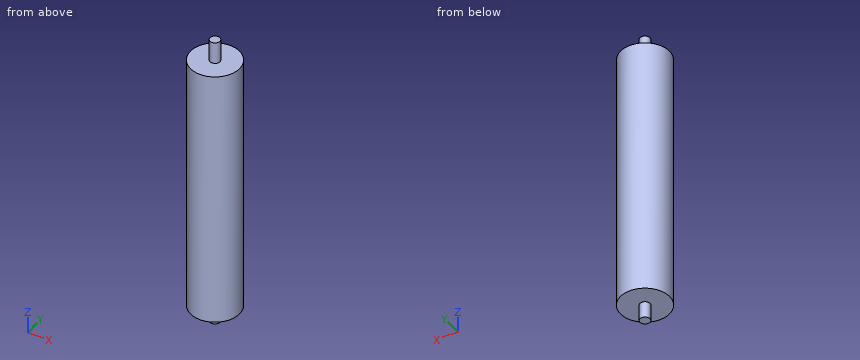
Autodesk Inventor part; units mm, degrees
ref_plane "YZ Plane" through (0, 0, 0) normal (1, 0, 0) x (0, 1, 0)
ref_plane "XZ Plane" through (0, 0, 0) normal (0, 1, 0) x (-1, 0, 0)
ref_plane "XY Plane" through (0, 0, 0) normal (0, 0, 1) x (1, 0, 0)
sketch "草图1" plane through (0, 0, 0) normal (0, 0, 1) x (1, 0, 0)
  circle A0 centre (0, 0) radius 4.6
  dimension "d0" = 9.2
extrude "拉伸1" add sketch "草图1" along normal blind 20
sketch "草图2" plane through (0, 0, 0) normal (0, 0, -1) x (-1, 0, 0)
  circle A0 centre (0, 0) radius 4.6
  circle A1 centre (0, 0) radius 22.5
  dimension "d3" = 45
extrude "拉伸2" add sketch "草图2" along normal blind 240 contours A0 | A1
sketch "草图3" plane through (0, 0, -240) normal (0, 0, -1) x (-1, 0, 0)
  circle A0 centre (0, 0) radius 4.6
  circle A1 centre (0, 0) radius 4.6
extrude "拉伸3" add sketch "草图3" along normal blind 15
properties part number "滚轴2"
Can you work these out from the model? Positions are in its coordinate system, mm. Coordinates: 2 decimals unless noted, no trailing zeros. Loops run counter-clockwise (first coordinate to the right, second up) from the corner with the lowest first, then second, coordinate; pieces in that order, holes last. Notation, with made-up numbers: (-17.75, 13) - (31.25, 13) arc R19 cw to (31.25, 35) - close; hole circle Ø6 at (60.5, 28.25). An arc over 180 degrees is marked (long way). Answer as CSV lines item,"result". Start each with the question number.
1) Suppose I cut it at D-D (y = 18). Please give me the cut outline in (x, z).
2) Suppose I cut it at C-C (z = -209.5). Please give me the cut outline in (x, y).
3) I need wall thicknesses on line 1 (Z direction, x = -2.5, y = -10); line 2 (Y direction, x = -20, z = -147); line 3 (Y direction, x = -5.5, z = -155.5). Which ranges of each line are inside material? Lowest first, please. Write a range as from..to.
4) Suppose I cut it at A-A (y = 0). Please give me the cut outline in (x, z).
5) For pin 1 (3 mm diameter, centred on x = 1.5, y = -13, fed in from -Z); pin 2 (4 mm diameter, centred on y = 4, z = -219, fed in from -X); pin 3 (10 mm diameter, centred on x = 18, y = 14.5, fed in from +Z), each with a flat end and sliding along its axis, tell me the tip position at first contact or that it passes through.
Check result:
1,outline,"(-13.5, -240) - (13.5, -240) - (13.5, 0) - (-13.5, 0) - close"
2,outline,"circle Ø45 at (0, 0)"
3,line 1,"z = -240..0"
3,line 2,"y = -10.31..10.31"
3,line 3,"y = -21.82..21.82"
4,outline,"(-22.5, -240) - (-4.6, -240) - (-4.6, -255) - (4.6, -255) - (4.6, -240) - (22.5, -240) - (22.5, 0) - (4.6, 0) - (4.6, 20) - (-4.6, 20) - (-4.6, 0) - (-22.5, 0) - close"
5,pin 1,"stops at z = -240"
5,pin 2,"stops at x = -22.41"
5,pin 3,"stops at z = 0"
